from build123d import *

# Parameters (mm, degrees)
F0_W     = 45
F0_H     = 45
F1_DEPTH = 10
F3_DEPTH = 10
F5_DEPTH = 10
F7_DEPTH = 10
F9_DEPTH = 10


with BuildPart() as f1:
    # F0 (on Top) → F1 (new body)
    with BuildSketch(Plane.XY):
        Rectangle(F0_W, F0_H)
    extrude(amount=F1_DEPTH)

    # F2 (on Top) → F3 (join)
    with BuildSketch(Plane.XY):
        Polygon((-21.650635, 22.5), (21.650635, 22.5), (-1.732051, 60.948017), align=None)
    extrude(amount=F3_DEPTH)

    # F4 (on Top) → F5 (join)
    with BuildSketch(Plane.XY):
        Polygon((22.5, -21.292087), (59.378976, 0), (22.5, 21.292087), align=None)
    extrude(amount=F5_DEPTH)

    # F6 (on Top) → F7 (join)
    with BuildSketch(Plane.XY):
        Polygon((-22.5, -22.5), (0, -61.471143), (22.5, -22.5), align=None)
    extrude(amount=F7_DEPTH)

    # F8 (on Top) → F9 (join)
    with BuildSketch(Plane.XY):
        Polygon((-22.5, 20.278981), (-57.624225, 0), (-22.5, -20.278981), align=None)
    extrude(amount=F9_DEPTH)


solid = f1.part
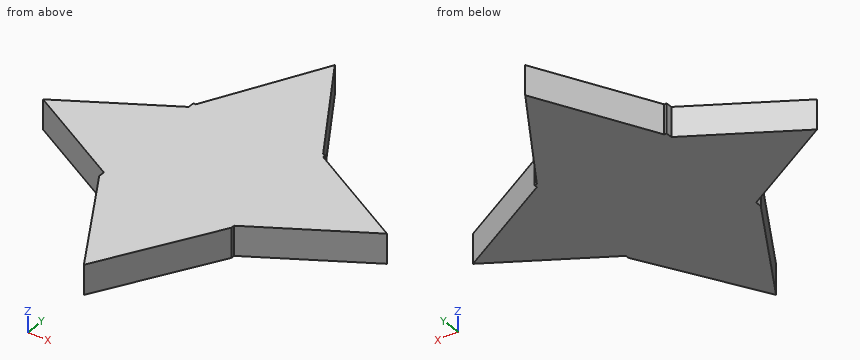
Could you check a few things on this model? Use its own coordinates, in mm. Give positions to 0.01 mm unless a question says otherwise; leave off trailing zeros. Write each loop counter-clockwise with the first axis right and the second up, starting at its lowest first coordinate (ties: lowest second). Pieces come first, ordered by that corner, then holes. Notation, with made-up numbers: (82, 31.5) -> (101, 31.5) arc R25 cw to (101, 49.5) -> close; hole circle Ø5 at (-3, 3.25). An arc over 180 degrees is marked (long way). Answer as a JSON object with one key per item and string values.
Q1. Please list where these lines run through material, in increasing order: L1, parallel to X at y = -24, z = 9; L2, parallel to Y at x = 7, z = 6.5; L3, parallel to X at y = -15, z = 2.
Taken from the geometry:
{"L1": "x = -21.63 to 21.63", "L2": "y = -49.35 to 46.59", "L3": "x = -31.64 to 33.4"}
Q2. Suppose I cut it at B-B on x = 9. Write out the boundary of the cut face in (y, z), then the cut area to 3 significant figures.
Taken from the geometry:
{"outline": "(-45.88, 0) -> (43.3, 0) -> (43.3, 10) -> (-45.88, 10) -> close", "area": "892 mm²"}
Q3. Suppose I cut it at C-C on y = 3. Write out the boundary of the cut face in (x, z).
Taken from the geometry:
{"outline": "(-52.43, 0) -> (54.18, 0) -> (54.18, 10) -> (-52.43, 10) -> close"}
Q4. Suppose I cut it at A-A on z = 5.25. Write out the boundary of the cut face in (x, y).
Taken from the geometry:
{"outline": "(-57.62, 0) -> (-22.5, -20.28) -> (-22.5, -22.5) -> (0, -61.47) -> (22.5, -22.5) -> (22.5, -21.29) -> (59.38, 0) -> (22.5, 21.29) -> (22.5, 22.5) -> (21.65, 22.5) -> (-1.73, 60.95) -> (-21.65, 22.5) -> (-22.5, 22.5) -> (-22.5, 20.28) -> close"}
Q5. Will these pins go through, and if not, where does the flat tip stop? pin 1 Ø3 at (y, z) = (-41.5, 8) entering from +X; pin 2 Ø1.3 at (y, z) = (-22, 7) entering from +X; pin 3 Ø1.8 at (y, z) = (21.5, 6.5) entering from -X.
Taken from the geometry:
{"pin 1": "stops at x = 12.4", "pin 2": "stops at x = 22.5", "pin 3": "stops at x = -22.5"}
